```python
from build123d import *

# Parameters (mm, degrees)
BOSS_EXTRUDE1_DEPTH                     = 20
CUT_EXTRUDE1_DEPTH                      = 20
CBORE_FOR_M5_HEX_HEAD_BOLT1_D           = 7.5
CBORE_FOR_M5_HEX_HEAD_BOLT1_DEPTH       = 112.583668517
CBORE_FOR_M5_HEX_HEAD_BOLT1_CBORE_D     = 11.25
CBORE_FOR_M5_HEX_HEAD_BOLT1_CBORE_DEPTH = 1.25
CBORE_FOR_M5_HEX_HEAD_BOLT1_TIP         = 2.253227321
CUT_EXTRUDE2_DEPTH                      = 10
SKETCH6_W                               = 20
SKETCH6_H                               = 20
BOSS_EXTRUDE2_DEPTH                     = 2.5
FILLET1_R                               = 2
FILLET2_R                               = 20
CUT_EXTRUDE3_DEPTH                      = 4.5
HOLE1_OUTLINE_R                         = 1.25
HOLE1_DEPTH                             = 2
LPATTERN1_COUNT                         = 3
LPATTERN1_PITCH                         = 6.8
LPATTERN1_COUNT_DIR2                    = 2
LPATTERN1_PITCH_DIR2                    = 12.5
LPATTERN2_COUNT                         = 2
LPATTERN2_PITCH                         = 29.6
LPATTERN2_COUNT_DIR2                    = 2
LPATTERN2_PITCH_DIR2                    = 12.5


# Read off the part's stored shape, not the designer's step: Hole1
with BuildPart() as part:
    # Sketch1 → Boss-Extrude1 (new body)
    with BuildSketch(Plane(origin=(0, 0, 0), x_dir=(1, 0, 0), z_dir=(0, 1, 0))):
        Polygon((29, 50.229473419), (0, 0), (130, 0), (130, 10), (78.679491924, 10), (25.732050808, 40.569219382), (30.732050808, 49.229473419), align=None)
    extrude(amount=BOSS_EXTRUDE1_DEPTH)

    # Sketch2 → Cut-Extrude1 (cut)
    with BuildSketch(Plane(origin=(0, 20, 0), x_dir=(1, 0, 0), z_dir=(0, 1, 0))):
        with BuildLine():
            Line((29.875644347, 2), (69.875644347, 2))
            ThreePointArc((69.875644347, 2), (74.705273478, 5.705904774), (72.375644347, 11.330127019))
            Line((72.375644347, 11.330127019), (29.062177826, 36.337168574))
            ThreePointArc((29.062177826, 36.337168574), (25.268082601, 36.836670687), (22.232050808, 34.507041555))
            Line((22.232050808, 34.507041555), (12.232050808, 17.186533479))
            ThreePointArc((12.232050808, 17.186533479), (11.732548695, 13.392438254), (14.062177826, 10.356406461))
            Line((14.062177826, 10.356406461), (27.375644347, 2.669872981))
            ThreePointArc((27.375644347, 2.669872981), (28.581549122, 2.170370869), (29.875644347, 2))
        make_face()
    extrude(amount=-CUT_EXTRUDE1_DEPTH, mode=Mode.SUBTRACT)

    # CBORE for M5 Hex Head Bolt1
    with Locations(Plane(origin=(0, 0, 0), x_dir=(-0.5000000000000042, 0, 0.8660254037844363), z_dir=(-0.8660254037844362, 0, -0.5000000000000041))):
        with Locations((-8, 10)):
            CounterBoreHole(CBORE_FOR_M5_HEX_HEAD_BOLT1_D / 2, CBORE_FOR_M5_HEX_HEAD_BOLT1_CBORE_D / 2, CBORE_FOR_M5_HEX_HEAD_BOLT1_CBORE_DEPTH, depth=CBORE_FOR_M5_HEX_HEAD_BOLT1_DEPTH)
            with Locations((0, 0, -(CBORE_FOR_M5_HEX_HEAD_BOLT1_DEPTH + CBORE_FOR_M5_HEX_HEAD_BOLT1_TIP / 2))):  # 118° drill point
                Cone(0, CBORE_FOR_M5_HEX_HEAD_BOLT1_D / 2, CBORE_FOR_M5_HEX_HEAD_BOLT1_TIP, mode=Mode.SUBTRACT)

    # Sketch5 → Cut-Extrude2 (cut)
    with BuildSketch(Plane.XY):
        with BuildLine():
            Line((95, 20), (130, 20))
            Line((130, 20), (130, 15))
            Line((130, 15), (98.75, 15))
            ThreePointArc((98.75, 15), (96.098349571, 16.098349571), (95, 18.75))
            Line((95, 18.75), (95, 20))
        make_face()
        with BuildLine():
            Line((95, 0), (130, 0))
            Line((130, 0), (130, 5))
            Line((130, 5), (98.75, 5))
            ThreePointArc((98.75, 5), (96.098349571, 3.901650429), (95, 1.25))
            Line((95, 1.25), (95, 0))
        make_face()
        with BuildLine():
            Line((130, 12.5), (112.5, 12.5))
            ThreePointArc((112.5, 12.5), (110, 10), (112.5, 7.5))
            Line((112.5, 7.5), (130, 7.5))
            Line((130, 7.5), (130, 12.5))
        make_face()
    extrude(amount=-CUT_EXTRUDE2_DEPTH, mode=Mode.SUBTRACT)

    # Sketch6 → Boss-Extrude2 (add)
    with BuildSketch(Plane(origin=(24, 0, -41.569219382), x_dir=(-0.8660254037844363, 0, -0.5000000000000042), z_dir=(0.5000000000000042, 0, -0.8660254037844363))):
        with Locations((-32, 10)):
            Rectangle(SKETCH6_W, SKETCH6_H)
    extrude(amount=BOSS_EXTRUDE2_DEPTH)

    # Fillet1
    fillet1_edges = [part.edges().sort_by_distance(p)[0] for p in [
        (60.373066959, 10, -20.569219382),
        (43.052558883, 10, -30.569219382),
        (25.732050808, 10, -40.569219382),
    ]]
    fillet(fillet1_edges, radius=FILLET1_R)

    # Fillet2
    fillet2_edges = [part.edges().sort_by_distance(p)[0] for p in [
        (78.679491924, 10, -10),
    ]]
    fillet(fillet2_edges, radius=FILLET2_R)

    # Sketch7 → Cut-Extrude3 (cut)
    with BuildSketch(Plane(origin=(25.25, 0, -43.734282891), x_dir=(-0.8660254037844363, 0, -0.5000000000000042), z_dir=(0.5000000000000042, 0, -0.8660254037844363))):
        with BuildLine():
            Line((-35.75, 13.75), (-28.25, 13.75))
            ThreePointArc((-28.25, 13.75), (-24.5, 10), (-28.25, 6.25))
            Line((-28.25, 6.25), (-35.75, 6.25))
            ThreePointArc((-35.75, 6.25), (-39.5, 10), (-35.75, 13.75))
        make_face()
    extrude(amount=-CUT_EXTRUDE3_DEPTH, mode=Mode.SUBTRACT)

    # Hole1 outline → Hole1 (cut)
    with BuildSketch(Plane(origin=(0, 0, 0), x_dir=(0.500000000000004, 0, -0.8660254037844363), z_dir=(0.8660254037844363, 0, 0.5000000000000042))):
        with Locations((24.5, 16.25)):
            Circle(HOLE1_OUTLINE_R)
    hole1 = extrude(amount=HOLE1_DEPTH, mode=Mode.SUBTRACT)

    # LPattern1: Hole1 3 × 2
    with Locations(*[Vector(0.5000000000000041, 0, -0.8660254037844363) * (i * LPATTERN1_PITCH) + Vector(0, -1, 0) * (j * LPATTERN1_PITCH_DIR2) for i in range(LPATTERN1_COUNT) for j in range(LPATTERN1_COUNT_DIR2) if (i, j) != (0, 0)]):
        add(hole1, mode=Mode.SUBTRACT)

    # LPattern2: Hole1 2 × 2, 1 skipped
    with Locations(*[Vector(0.5000000000000041, 0, -0.8660254037844363) * (i * LPATTERN2_PITCH) + Vector(0, -1, 0) * (j * LPATTERN2_PITCH_DIR2) for i in range(LPATTERN2_COUNT) for j in range(LPATTERN2_COUNT_DIR2) if (i, j) not in ((0, 0), (0, 1))]):
        add(hole1, mode=Mode.SUBTRACT)


solid = part.part
```
For this review, take the finished solid that the model builds, in its own axes (mm). A direction names the side the tool comes from. Round coordinates to 2 decimals unless told otherwise and drop trailing zeros. Write each loop counter-clockwise with the first axis right and the second up, starting at its lowest first coordinate (ties: lowest second). Pieces come first, ordered by that corner, then holes. Notation, with made-up numbers: (30.5, 54.5) -> (70.5, 54.5) arc R32 ccw to (70.5, 91.5) -> close; hole circle Ø5 at (39.5, 79). An arc over 180 degrees is marked (long way). Use one line per item in the form item = value.
Q1. Consider section B-B (x = 33). State the section outline as (y, z) points.
Resolved:
outline = (0, -36.37) -> (20, -36.37) -> (20, -34.06) -> (0, -34.06) -> close; (0, -2) -> (20, -2) -> (20, 0) -> (0, 0) -> close
Q2. The part is to be moulded in two halves that separate along X. For faces 1 (the flat face through (115, 15, -5)), 2 (the flat face through (68.155, 9.86, -16.076)), 3 (the cylindrical face through (25.32, 10.14, -36.85)), say which applies: released by +X, released by -X, zero draft, split by the parting line, or undercut.
Resolved:
face_1 = zero draft
face_2 = released by +X
face_3 = undercut
Q3. Clearance check with flat-ended pins moving along their axes: pin 1 Ø1.5 at (y, z) = (17.5, -29) entering from -X; pin 2 Ø10 at (x, y) = (118.5, 14) entering from -Z; pin 3 Ø1.4 at (y, z) = (19.5, -6.5) entering from +X; pin 4 Ø4 at (x, z) = (50.5, -24.5) entering from -Y. State where each tip first meets the part, or that it passes through.
Resolved:
pin_1 = 16.31
pin_2 = -10
pin_3 = 95
pin_4 = 0
Q4. Consider section C-C (x = 97.5). State the section outline as (y, z) points, then the cut area to 3 significant figures.
Resolved:
outline = (4.79, -10) -> (15.21, -10) -> (15.21, 0) -> (4.79, 0) -> close
area = 104 mm²
Q5. To check wall thickness, follow probe 1 along Y at (x, z) = (54.5, -24.5); probe 2 along Z at (x, y) = (93.5, 14.5); probe 3 along Z at (x, y) = (25.5, 17.5). State the ranges of each line that lie inside material, in increasing order. Write a range as from..to.
Resolved:
probe_1 = 0..6.25, 13.75..20
probe_2 = -10..0
probe_3 = -44.17..-36.89, -3.75..0
Q6. Machinability: for faces 4 (the flat face through (50, 10, -2)), 5 (the cylindrical face through (45.359, 10.082, -29.563)), 6 (the flat face through (121, 12.5, -5)), 7 (the cylindrical face through (42.817, 10.14, -31.364)), 8 (the flat face through (52, 6.25, -26)), which of the approach directions +Z, -Z, +X, -X, +Y, -Y give a long, thin tool a straight path to every point of the face, cutting with its end or side? Answer none if there is none.
Resolved:
face_4 = +Y, -Y
face_5 = +X
face_6 = +Z, -Z, +X
face_7 = -Z, +Y, -Y
face_8 = none
Q7. Consider section A-A (x = 122). State the section outline as (y, z) points.
Resolved:
outline = (5, -10) -> (7.5, -10) -> (7.5, 0) -> (5, 0) -> close; (12.5, -10) -> (15, -10) -> (15, 0) -> (12.5, 0) -> close
